Can you work these out from the model? Positions are in its coordinate system, mm. Face numbers are marked on the shaded views. A direction names the side the tool comes from. Round coordinates to 2 decimals unless told otherwise and drop trailing zeros. Loops run counter-clockwise (first coordinate to the right, second up) from the corner with the lowest first, then second, coordinate; pieces in that order, holes last.
(1) If I drill on line 1 along Y through (x, z) = (21.55, 1.65); line 2 along X through (y, z) = (20.5, 6.5); line 3 along X through (y, z) = (-21, 1.5), over which ranges is the centre line in solid material (lowest first)?
(2) I want a section at A-A on y = -10.5. Write out the boundary of the cut face in (x, z), plus the area to 3 significant figures.
(3) Which directions (+Z, -Z, +X, -X, +Y, -Y) give clear straight access to the entire face, cutting with the end or side of a thin tool? Please do the marked faces 1 and 2.
(4) I want a section at D-D on x = -102. Write out the boundary of the cut face in (y, z), plus the area to 3 significant figures.
(5) I want a section at B-B on z = 16.5. Write out the boundary of the cut face in (x, y), plus the area to 3 significant figures.
(6) I want a section at C-C on x = 21.55. Write out the boundary of the cut face in (y, z).
(7) Will these pins go through, and if not, where does the flat tip stop? pin 1 Ø12 at (x, y) = (138.5, 1) entering from +Z; pin 2 Ø3.5 at (x, y) = (21.55, -21.55) entering from +Z; pin 3 Ø8 at (y, z) = (-1, 16.5) entering from +X; pin 4 Ø1.5 at (y, z) = (21, 15) entering from -X.
from build123d import *

# Parameters (mm, degrees)
SKETCH1_W           = 330
SKETCH1_H           = 56.2
BOSS_EXTRUDE1_DEPTH = 10
SKETCH2_W           = 56.2
SKETCH2_H           = 56.2
CUT_EXTRUDE1_DEPTH  = 5
SKETCH3_W           = 10
SKETCH3_H           = 56.2
BOSS_EXTRUDE2_DEPTH = 10
SKETCH4_W           = 10
SKETCH4_H           = 56.2
BOSS_EXTRUDE3_DEPTH = 10
CUT_EXTRUDE2_DEPTH  = 56.2
SKETCH6_W           = 10
SKETCH6_H           = 56.2
BOSS_EXTRUDE4_DEPTH = 10
SKETCH7_W           = 10
SKETCH7_H           = 56.2
BOSS_EXTRUDE5_DEPTH = 10
CUT_EXTRUDE3_DEPTH  = 56.2
SKETCH9_W           = 30
SKETCH9_H           = 30
CUT_EXTRUDE4_DEPTH  = 5
SKETCH10_R          = 3
CUT_EXTRUDE5_DEPTH  = 5


with BuildPart() as part:
    # Sketch1 → Boss-Extrude1 (new body)
    with BuildSketch(Plane.XY):
        Rectangle(SKETCH1_W, SKETCH1_H)
    extrude(amount=BOSS_EXTRUDE1_DEPTH)

    # Sketch2 → Cut-Extrude1 (cut)
    with BuildSketch(Plane.XY.offset(10)):
        Rectangle(SKETCH2_W, SKETCH2_H)
    extrude(amount=-CUT_EXTRUDE1_DEPTH, mode=Mode.SUBTRACT)

    # Sketch3 → Boss-Extrude2 (add)
    with BuildSketch(Plane(origin=(165, 0, 0), x_dir=(0, 0, -1), z_dir=(1, 0, 0))):
        with Locations((-5, 0)):
            Rectangle(SKETCH3_W, SKETCH3_H)
    extrude(amount=BOSS_EXTRUDE2_DEPTH)

    # Sketch4 → Boss-Extrude3 (add)
    with BuildSketch(Plane.XY.offset(10)):
        with Locations((170, 0)):
            Rectangle(SKETCH4_W, SKETCH4_H)
    extrude(amount=BOSS_EXTRUDE3_DEPTH)

    # Sketch5 → Cut-Extrude2 (cut)
    with BuildSketch(Plane(origin=(0, 28.1, 0), x_dir=(1, 0, 0), z_dir=(0, 1, 0))):
        Polygon((165, -20), (175, -10), (175, -20), align=None)
    extrude(amount=-CUT_EXTRUDE2_DEPTH, mode=Mode.SUBTRACT)

    # Sketch6 → Boss-Extrude4 (add)
    with BuildSketch(Plane.ZY.offset(165)):
        with Locations((5, 0)):
            Rectangle(SKETCH6_W, SKETCH6_H)
    extrude(amount=BOSS_EXTRUDE4_DEPTH)

    # Sketch7 → Boss-Extrude5 (add)
    with BuildSketch(Plane.XY.offset(10)):
        with Locations((-170, 0)):
            Rectangle(SKETCH7_W, SKETCH7_H)
    extrude(amount=BOSS_EXTRUDE5_DEPTH)

    # Sketch8 → Cut-Extrude3 (cut)
    with BuildSketch(Plane(origin=(0, 28.1, 0), x_dir=(1, 0, 0), z_dir=(0, 1, 0))):
        Polygon((-165, -20), (-175, -10), (-175, -20), align=None)
    extrude(amount=-CUT_EXTRUDE3_DEPTH, mode=Mode.SUBTRACT)

    # Sketch9 → Cut-Extrude4 (cut)
    with BuildSketch(Plane.XY.offset(5)):
        Rectangle(SKETCH9_W, SKETCH9_H)
    extrude(amount=-CUT_EXTRUDE4_DEPTH, mode=Mode.SUBTRACT)

    # Sketch10 → Cut-Extrude5 (cut)
    with BuildSketch(Plane.XY.offset(5)):
        with Locations((-21.55, 21.55)):
            Circle(SKETCH10_R)
        with Locations((21.55, -21.55)):
            Circle(SKETCH10_R)
    extrude(amount=-CUT_EXTRUDE5_DEPTH, mode=Mode.SUBTRACT)


solid = part.part
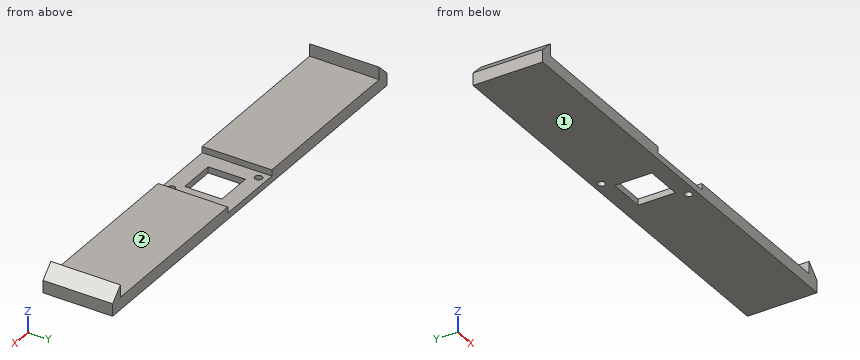
Filled sheet:
1. line 1: y = -28.1 to -24.55, -18.55 to 28.1
1. line 2: x = -175 to -28.1, 28.1 to 175
1. line 3: x = -175 to 18.6, 24.5 to 175
2. outline: (-175, 0) - (-15, 0) - (-15, 5) - (-28.1, 5) - (-28.1, 10) - (-165, 10) - (-165, 20) - (-175, 10) - close; (15, 0) - (175, 0) - (175, 10) - (165, 20) - (165, 10) - (28.1, 10) - (28.1, 5) - (15, 5) - close
2. area: 3,170 mm2
3. face 1: -Z, +X, -X, +Y, -Y
3. face 2: +Z, +Y, -Y
4. outline: (-28.1, 0) - (28.1, 0) - (28.1, 10) - (-28.1, 10) - close
4. area: 562 mm2
5. outline: (-168.5, -28.1) - (-165, -28.1) - (-165, 28.1) - (-168.5, 28.1) - close; (165, -28.1) - (168.5, -28.1) - (168.5, 28.1) - (165, 28.1) - close
5. area: 393 mm2
6. outline: (-28.1, 0) - (-24.55, 0) - (-24.55, 5) - (-28.1, 5) - close; (-18.55, 0) - (28.1, 0) - (28.1, 5) - (-18.55, 5) - close
7. pin 1: stops at z = 10
7. pin 2: passes through
7. pin 3: stops at x = 172.5
7. pin 4: stops at x = -170.75
